Here's the drawing with two shaded views (mm, measured from the low corner). I have some questions. Give positions to 0.01 mm unless a question says otherwise; leave off trailing zeros. Loops run counter-clockwise (first coordinate to the right, second up) from the corner with the lowest first, then second, coordinate; pieces in that order, holes last.
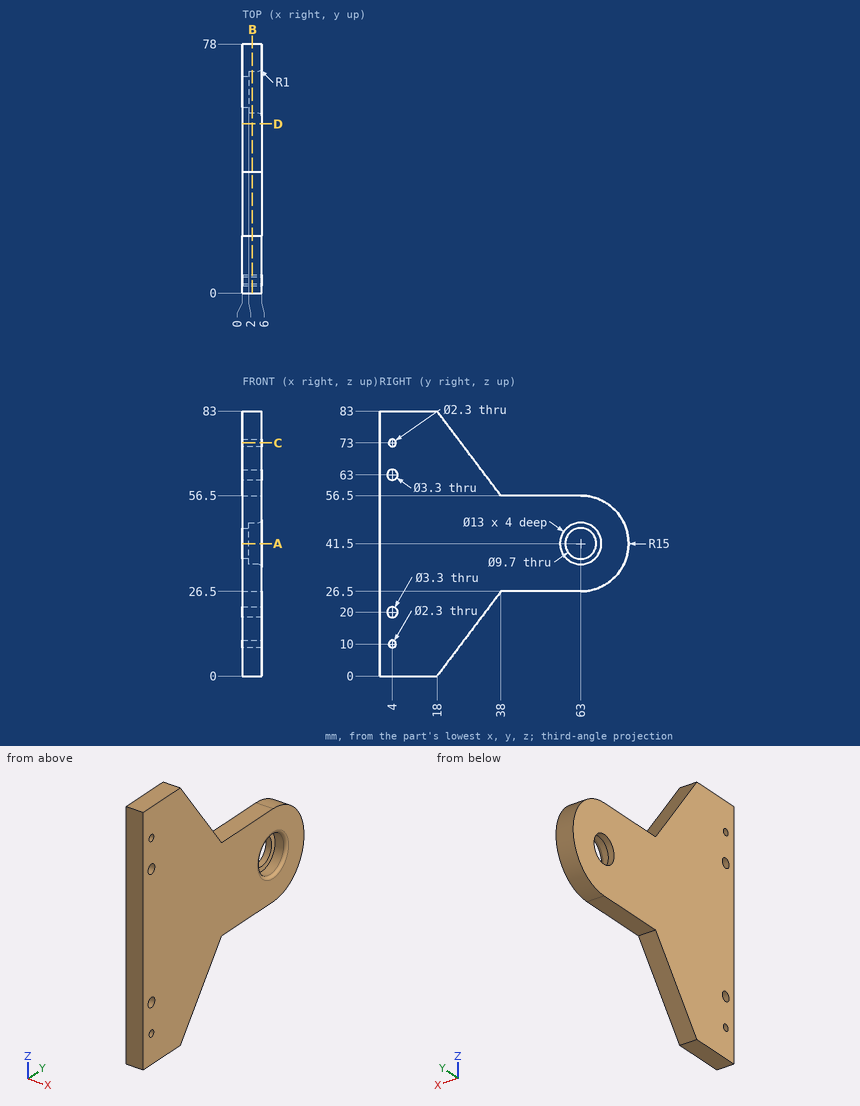
(1) Suppose I cut it at C-C on z = 73. List the corners of the cut face in (x, y) for me, plus the area to 3 significant figures.
Returned:
outline: (0, 0) - (6, 0) - (6, 2.85) - (0, 2.85) - close; (0, 5.15) - (6, 5.15) - (6, 25.55) - (0, 25.55) - close
area: 139 mm2
(2) Suppose I cut it at D-D on y = 53. List the corners of the cut face in (x, z) for me.
Returned:
outline: (0, 26.5) - (6, 26.5) - (6, 56.5) - (0, 56.5) - close
(3) Suppose I cut it at A-A on z = 41.5. List the corners of the cut face in (x, y) for me.
Returned:
outline: (0, 0) - (6, 0) - (6, 55.5) arc R1 ccw to (5, 56.5) - (2, 56.5) - (2, 58.15) - (0, 58.15) - close; (0, 67.85) - (2, 67.85) - (2, 69.5) - (5, 69.5) arc R1 ccw to (6, 70.5) - (6, 78) - (0, 78) - close
(4) Suppose I cut it at B-B on x = 3.1. List the corners of the cut face in (y, z) for me, plus the area to 3 significant figures.
Returned:
outline: (0, 0) - (18, 0) - (38, 26.5) - (63, 26.5) arc R15 ccw to (63, 56.5) - (38, 56.5) - (18, 83) - (0, 83) - close; hole circle Ø3.3 at (4, 20); hole circle Ø3.3 at (4, 63); hole circle Ø2.3 at (4, 10); hole circle Ø2.3 at (4, 73); hole circle Ø13 at (63, 41.5)
area: 3,570 mm2
(5) Will these pins go through, and if not, where does the flat tip stop? P1, Ø3, axis at y = 4, z = 63, coming from the +X side; P2, Ø2, axis at x = 5, y = 34.5, coming from the +Z side; P3, Ø2, axis at x = 2, y = 67, coming from the -Z side; P4, Ø3, axis at x = 2, y = 42, coming from the +Z side.
Returned:
P1: passes through
P2: stops at z = 62.46
P3: stops at z = 26.8
P4: stops at z = 56.5
(6) Please list where these lines run through material, in increasing order: probe 1 along Y at (x, z) = (1.7, 63); probe 2 along Y at (x, z) = (5.7, 45.5); probe 3 along Z at (x, y) = (5.1, 44).
Returned:
probe 1: y = 0 to 2.35, 5.65 to 33.09
probe 2: y = 0 to 57.52, 68.48 to 77.46
probe 3: z = 26.5 to 56.5
